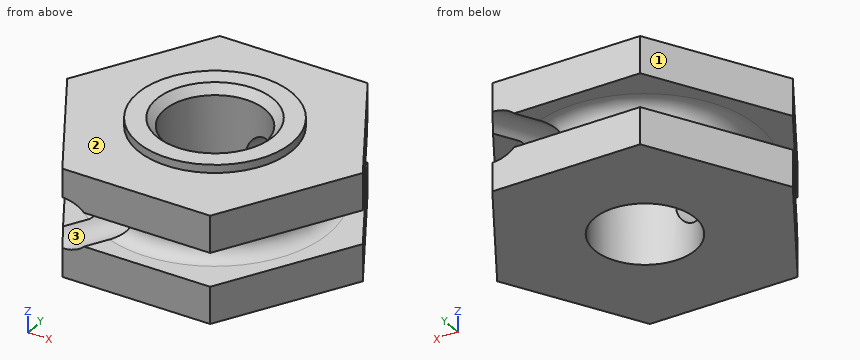
Autodesk Inventor part; units mm, degrees
ref_plane "Work Plane1" through (3.4829, 6.0325, 0) normal (0.5, 0.866, 0) x (0, 0, 1)
ref_plane "Work Plane2" through (3.4829, 6.0325, 0) normal (0.866, -0.5, 0) x (0, 0, 1)
ref_plane "YZ Plane" through (0, 0, 0) normal (1, 0, 0) x (0, 1, 0)
sketch "Sketch1" plane through (0, 0, 0) normal (0, 0, 1) x (1, 0, 0)
  circle A0 centre (0, 0) radius 6.0325 construction
  line L0 (3.4829, 6.0325) -> (6.9657, 0)
  line L1 (6.9657, 0) -> (3.4829, -6.0325)
  line L2 (3.4829, -6.0325) -> (-3.4829, -6.0325)
  line L3 (-3.4829, -6.0325) -> (-6.9657, 0)
  line L4 (-6.9657, 0) -> (-3.4829, 6.0325)
  line L5 (-3.4829, 6.0325) -> (3.4829, 6.0325)
  point P0 (0, 6.0325)
  dimension "d0" = 12.065
extrude "Extrusion1" add sketch "Sketch1" along normal mid plane 5.08
sketch "Sketch2" plane through (0, 0, 2.54) normal (0, 0, 1) x (1, 0, 0)
  circle A0 centre (0, 0) radius 2.3813
  circle A1 centre (0, 0) radius 3.6513
  dimension "d3" = 4.7625
  dimension "d4" = 1.27
extrude "Extrusion2" add sketch "Sketch2" along normal blind 0.381
extrude "Extrusion3" cut sketch "Sketch2" against normal through all contours A0
chamfer "Chamfer1" distance 0.381 angle 45 1 edges at (-2.3813, 0, 2.921)
ref_plane "Work Plane1" through (3.4829, 6.0325, 0) normal (0.5, 0.866, 0) x (0, 0, 1)
sketch "Sketch3" plane through (3.4829, 6.0325, 0) normal (0.5, 0.866, 0) x (0, 0, 1)
  circle A0 centre (0, 0) radius 1.1913
  dimension "d13" = 2.3825
extrude "Extrusion4" cut sketch "Sketch3" against normal through all
ref_plane "Work Plane2" through (3.4829, 6.0325, 0) normal (0.866, -0.5, 0) x (0, 0, 1)
sketch "Sketch4" plane through (3.4829, 6.0325, 0) normal (0.866, -0.5, 0) x (0, 0, 1)
  line L0 (-1.1913, 4.5845) -> (-1.1913, 0) construction
  line L1 (-1.1913, 0) -> (-2.54, 0) construction
  line L2 (-2.54, 0) -> (-2.54, 4.5845) construction
  line L3 (-2.54, 4.5845) -> (-1.1913, 4.5845) construction
  line L4 (-1.1913, 13.9315) -> (-1.1913, 9.347) construction
  line L5 (-1.1913, 9.347) -> (-2.54, 9.347) construction
  line L6 (-2.54, 9.347) -> (-2.54, 13.9315) construction
  line L7 (-2.54, 13.9315) -> (-1.1913, 13.9315) construction
  line L8 (2.921, 9.728) -> (2.54, 9.347) construction
  line L9 (2.54, 9.347) -> (1.1913, 9.347) construction
  line L10 (1.1913, 9.347) -> (1.1913, 13.9315) construction
  line L11 (1.1913, 13.9315) -> (2.54, 13.9315) construction
  line L12 (2.54, 13.9315) -> (2.54, 10.617) construction
  line L13 (2.54, 10.617) -> (2.921, 10.617) construction
  line L14 (2.921, 10.617) -> (2.921, 9.728) construction
  line L15 (2.54, 4.5845) -> (2.921, 4.2035) construction
  line L16 (2.921, 4.2035) -> (2.921, 3.3145) construction
  line L17 (2.921, 3.3145) -> (2.54, 3.3145) construction
  line L18 (2.54, 3.3145) -> (2.54, 0) construction
  line L19 (2.54, 0) -> (1.1913, 0) construction
  line L20 (1.1913, 0) -> (1.1913, 4.5845) construction
  line L21 (1.1913, 4.5845) -> (2.54, 4.5845) construction
  line L22 (-0.7937, 0) -> (-0.7937, 1.5875)
  arc A0 (0.7938, 1.5875) -> (-0.7937, 1.5875) centre (0, 1.5875) ccw
  line L23 (0.7938, 1.5875) -> (0.7938, 0)
  line L24 (0.7938, 0) -> (-0.7937, 0)
  line L25 (-3.6322, 6.9657) -> (4.0132, 6.9657)
  point P0 (0, 6.9657)
  dimension "d16" = 1.5875
  dimension "d17" = 1.5875
revolve "Revolution1" cut sketch "Sketch4" angle 360 about axis through (0, 0, -10) along (0, 0, 1)
equation "\"d17\" = d16"
properties part number "Hex Drive"
Here's how the part is built. I have some questions about the finished solid (model axes, mm). Face numbers are marked on the shaded views. Coordinates: 2 decimals unless noted, no trailing zeros. Order: outer loops, then holes, each group sorted by start corner. A loop starts at its lowest first (then second) coordinate and runs counter-clockwise, first axis right, second up.
Item 1: I'm going to push flat-ended pins straight in: pin 1 Ø3 at (x, y) = (5, 5) entering from +Z; pin 2 Ø1 at (x, y) = (-2, 1) entering from +Z; pin 3 Ø2 at (y, z) = (-2.5, -1.5) entering from +X. Where does each tip first touch, or does it pass through?
Response values:
pin 1: stops at z = 2.54
pin 2: stops at z = 2.9
pin 3: stops at x = 6.1
Item 2: If we section it at A-A, the plane z = 1.6: List the corners of the cut face in (x, y) for me, then the cut area to 3 significant figures.
Response values:
outline: (-6.97, 0) - (-3.48, -6.03) - (3.48, -6.03) - (6.97, 0) - (3.48, 6.03) - (-3.48, 6.03) - close; hole circle Ø4.76 at (0, 0)
area: 108 mm2
Item 3: Thinking about a two-plate mould opening in X: for the marked faces 1, 2 and 3, which applies, pulls with the +X half, pulls with the -X half, needs draft (parallel to the pull), parting line crosses it, or undercut?
Response values:
face 1: pulls with the -X half
face 2: needs draft
face 3: undercut
Item 4: I need wall thicknesses on probe 1 along Y at (x, z) = (0, -0.95); probe 2 along Z at (x, y) = (-3.5, 1.5); probe 3 along Z at (x, y) = (-5, 3.25). Which ranges of each line are inside material? Lowest first, please.
Response values:
probe 1: y = -6.03 to -2.38, 2.38 to 6.03
probe 2: z = -2.54 to 2.54
probe 3: z = -2.54 to -0.79, 0.79 to 2.54
